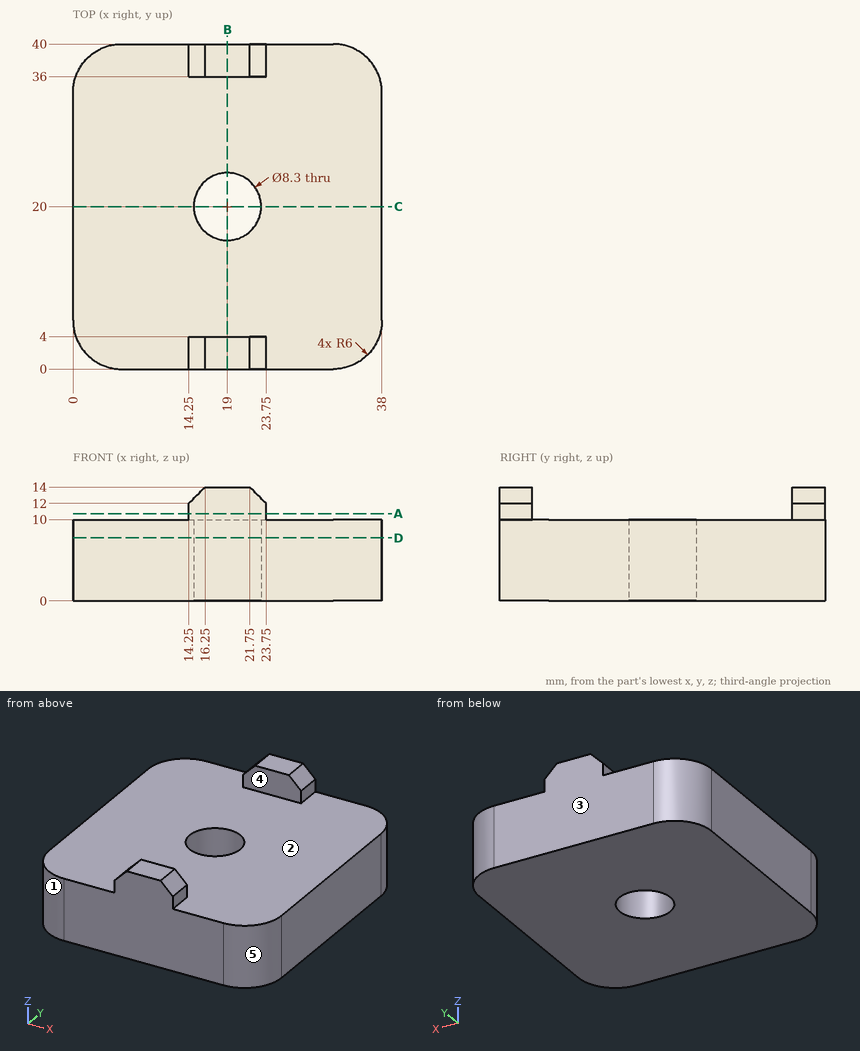
Verification items for this drawing (mm, ordinates from the low corner). A direction names the side the tool comes from. Give positions to 0.01 mm unless a question says otherwise; leave off trailing zeros. Order: outer loops, then holes, each group sorted by start corner. A loop starts at its lowest first (then second) coordinate and runs counter-clockwise, first axis right, second up.
1) Cross-section at B-B (x = 19). Record the boundary of the cut face in (y, z), then the cut area to 3 significant figures.
Results are:
outline: (0, 0) - (15.85, 0) - (15.85, 10) - (4, 10) - (4, 14) - (0, 14) - close; (24.15, 0) - (40, 0) - (40, 14) - (36, 14) - (36, 10) - (24.15, 10) - close
area: 349 mm2
2) Draft check along Y on the marked faces 1, 2 and 3. Enter one of: released by +Y, released by -Y, zero draft, split by the parting line, or undercut.
Results are:
face 1: released by -Y
face 2: undercut
face 3: released by +Y
3) Tool access check on the marked faces 4 and 5. Record the directions out of +Z, -Z, +X, -X, +Y, -Y that give a thin tool (end or side, any length) a straight path to the whole face; none if there is none.
Results are:
face 4: +Z, +X, -X
face 5: +Z, -Z, +X, -Y
4) Cross-section at C-C (y = 20). Record the boundary of the cut face in (x, z).
Results are:
outline: (0, 0) - (14.85, 0) - (14.85, 10) - (0, 10) - close; (23.15, 0) - (38, 0) - (38, 10) - (23.15, 10) - close
5) Gauge pin test, flat ends, axial feed: pin 1 (1 mm diameter, centred on x = 17, y = 33, fed in from +Z); pin 2 (1.6 mm diameter, centred on y = 37.5, z = 11, fed in from -X); pin 3 (0.6 mm diameter, centred on y = 39, z = 11.5, fed in from +X). Record the tip position at first contact, or that the pin passes through.
Results are:
pin 1: stops at z = 10
pin 2: stops at x = 14.25
pin 3: stops at x = 23.75
6) Cross-section at D-D (z = 7.75). Record the boundary of the cut face in (x, y), then the cut area to 3 significant figures.
Results are:
outline: (0, 6) arc R6 ccw to (6, 0) - (32, 0) arc R6 ccw to (38, 6) - (38, 34) arc R6 ccw to (32, 40) - (6, 40) arc R6 ccw to (0, 34) - close; hole circle Ø8.3 at (19, 20)
area: 1,430 mm2
7) Material ranges on probe 1 along Y at (x, z) = (19, 6.75); probe 2 along Y at (x, z) = (20, 13.75); probe 3 along Z at (x, y) = (33.5, 14), recorded low to high.
Results are:
probe 1: y = 0 to 15.85, 24.15 to 40
probe 2: y = 0 to 4, 36 to 40
probe 3: z = 0 to 10
8) Cross-section at A-A (z = 10.75). Record the boundary of the cut face in (x, y), then the cut area to 3 significant figures.
Results are:
outline: (14.25, 0) - (23.75, 0) - (23.75, 4) - (14.25, 4) - close; (14.25, 36) - (23.75, 36) - (23.75, 40) - (14.25, 40) - close
area: 76.0 mm2
